```python
from build123d import *

# Parameters (mm, degrees)
SKETCH1_W           = 353.187
SKETCH1_H           = 38.1
SKETCH1_R           = 8.911624301
BOSS_EXTRUDE1_DEPTH = 5.08
FILLET1_R           = 5.08


with BuildPart() as part:
    # Sketch1 → Boss-Extrude1 (new body)
    with BuildSketch(Plane(origin=(0, 0, 0), x_dir=(1, 0, 0), z_dir=(0, 1, 0))):
        Rectangle(SKETCH1_W, SKETCH1_H)
        with Locations(Location((0, 0, 0), (0, 0, 270))):
            Circle(SKETCH1_R, mode=Mode.SUBTRACT)
    extrude(amount=-BOSS_EXTRUDE1_DEPTH)

    # Fillet1
    fillet1_edges = [part.edges().sort_by_distance(p)[0] for p in [
        (-176.5935, -2.54, -19.05),
        (176.5935, -2.54, -19.05),
        (176.5935, -2.54, 19.05),
        (-176.5935, -2.54, 19.05),
    ]]
    fillet(fillet1_edges, radius=FILLET1_R)


solid = part.part
```
Part model, mm, in its own coordinate system. Coordinates: 2 decimals unless noted, no trailing zeros. Order: outer loops, then holes, each group sorted by start corner. A loop starts at its lowest first (then second) coordinate and runs counter-clockwise, first axis right, second up. Notation, with made-up numbers: (21, 54.25) -> (65, 54.25) arc R23 ccw to (65, 66.25) -> close; hole circle Ø5 at (-13.75, 4). An arc over 180 degrees is marked (long way). Put each result on its own line as item: value. Start each with the question number.
(1) Band-saw the part on A-A (z = 0). Give the cut face in (x, y).
(2) Mould opens along X. For faces 1 (the face through (-5.423, -2.504, -7.072)), 2 (the face through (-2, -5.08, -9)) say: pulls with the +X half, pulls with the -X half, needs draft (parallel to the pull), parting line crosses it, or undercut.
(3) Probe line 1 along X through (y, z) = (-2.5, 0); line 2 along X through (y, z) = (-4.6, -1.5); line 3 along X through (y, z) = (-2.7, -15). List the from-to ranges inside material, lowest first. Write a range as [from, to].
(4) Band-saw the part on C-C (y = -3.9). Give the cut face in (x, z), then the cut area to 3 significant figures.
(5) Band-saw the part on B-B (x = 0). Give the cut face in (y, z), then the cut area to 3 significant figures.
Determined:
1. outline: (-176.59, -5.08) -> (-8.91, -5.08) -> (-8.91, 0) -> (-176.59, 0) -> close; (8.91, -5.08) -> (176.59, -5.08) -> (176.59, 0) -> (8.91, 0) -> close
2. face 1: undercut
2. face 2: needs draft
3. line 1: x = [-176.59, -8.91], [8.91, 176.59]
3. line 2: x = [-176.59, -8.78], [8.78, 176.59]
3. line 3: x = [-176.49, 176.49]
4. outline: (-176.59, -13.97) arc R5.08 ccw to (-171.51, -19.05) -> (171.51, -19.05) arc R5.08 ccw to (176.59, -13.97) -> (176.59, 13.97) arc R5.08 ccw to (171.51, 19.05) -> (-171.51, 19.05) arc R5.08 ccw to (-176.59, 13.97) -> close; hole circle Ø17.82 at (0, 0)
4. area: 13,200 mm²
5. outline: (-5.08, -19.05) -> (0, -19.05) -> (0, -8.91) -> (-5.08, -8.91) -> close; (-5.08, 8.91) -> (0, 8.91) -> (0, 19.05) -> (-5.08, 19.05) -> close
5. area: 103 mm²
